The model under review builds one solid part; all positions refer to its coordinate system, in mm. Coordinates: 2 decimals unless noted, no trailing zeros. Loops run counter-clockwise (first coordinate to the right, second up) from the corner with the lowest first, then second, coordinate; pieces in that order, holes last. Notation, with made-up numbers: M 12,57 L 46,57 A31 ccw 46,92 Z; hole C 41.5,-16 d4. An arc over 180 degrees is marked long. Use one line per item in the form item = value.
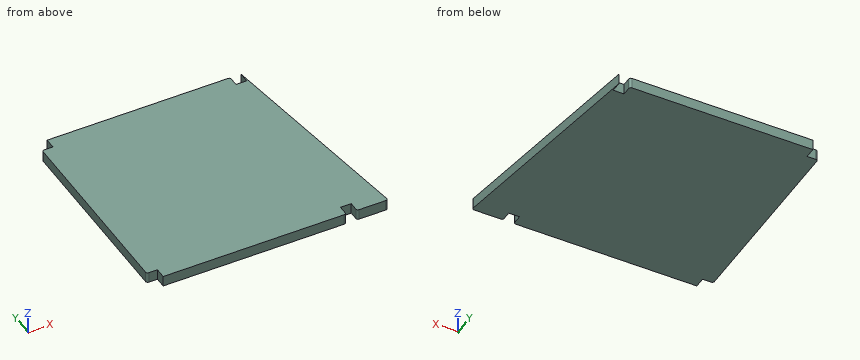
```python
from build123d import *

# Parameters (mm, degrees)
BOSS_EXTRUDE1_DEPTH = 5
FILLET1_R           = 1


with BuildPart() as part:
    # Sketch1 → Boss-Extrude1 (new body)
    with BuildSketch(Plane.XY):
        Polygon((0, 95.05), (0, 100), (85, 100), (85, 95.05), (90, 95.05), (90, 100), (104.5, 0), (90, 0), (90, 4.95), (85, 4.95), (85, 0), (0, 0), (0, 4.95), (-5, 4.95), (-5, 95.05), align=None)
    extrude(amount=BOSS_EXTRUDE1_DEPTH)

    # Fillet1
    fillet1_edges = [part.edges().sort_by_distance(p)[0] for p in [
        (-5, 4.95, 2.5),
        (-5, 95.05, 2.5),
        (85, 100, 2.5),
        (104.5, 0, 2.5),
        (90, 0, 2.5),
        (85, 0, 2.5),
    ]]
    fillet(fillet1_edges, radius=FILLET1_R)


solid = part.part
```
1. Add section A-A (z = 2.8). State the section outline as (x, y) points.
Response values:
outline = M -5,5.95 A1 ccw -4,4.95 L 0,4.95 L 0,0 L 84,0 A1 ccw 85,1 L 85,4.95 L 90,4.95 L 90,1 A1 ccw 91,0 L 103.34,0 A1 ccw 104.33,1.14 L 90,100 L 90,95.05 L 85,95.05 L 85,99 A1 ccw 84,100 L 0,100 L 0,95.05 L -4,95.05 A1 ccw -5,94.05 Z
2. Insertion check: P1, Ø1.5, axis at y = 97, z = 1.5, coming from the -X side; P2, Ø3, axis at x = -2, z = 1.5, coming from the -Y side; P3, Ø2, axis at y = 14.5, z = 1, coming from the +X side. Each pin has a flat end and moves straight along its axis. Give the tip position at first contact, or say it passes through.
Response values:
P1 = 0
P2 = 4.95
P3 = 102.54
3. Add section B-B (y = 74). State the section outline as (x, z) points.
Response values:
outline = M -5,0 L 93.77,0 L 93.77,5 L -5,5 Z
4. Add section C-C (y = 37). State the section outline as (x, z) points (3 decimals).
Response values:
outline = M -5,0 L 99.135,0 L 99.135,5 L -5,5 Z
5. Wall thickness on line 1 along X through (y, z) = (43.5, 2.8); line 2 along X through (y, z) = (39, 1.1) (3 decimals): over which ranges is each line inside the solid? List them lowest first. Write a range as from..to.
Response values:
line_1 = -5..98.19
line_2 = -5..98.845
